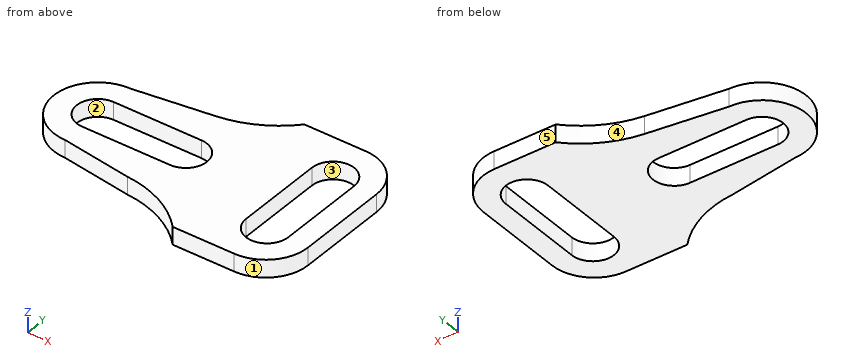
from build123d import *

# Parameters (mm, degrees)
BOSS_EXTRUDE1_DEPTH = 50


with BuildPart() as part:
    # Sketch1 → Boss-Extrude1 (new body)
    with BuildSketch(Plane.XY):
        with BuildLine():
            Line((-175, 353.543476539), (0, 353.543476539))
            ThreePointArc((0, 353.543476539), (84.852813742, 318.396290281), (120, 233.543476539))
            Line((120, 233.543476539), (120, -26.456523461))
            ThreePointArc((120, -26.456523461), (84.852813742, -111.309337204), (0, -146.456523461))
            Line((0, -146.456523461), (-175, -146.456523461))
            ThreePointArc((-175, -146.456523461), (-265.915006149, -79.830220617), (-375, -51.456523461))
            Line((-375, -51.456523461), (-575, -21.456523461))
            ThreePointArc((-575, -21.456523461), (-700, 103.543476539), (-575, 228.543476539))
            Line((-575, 228.543476539), (-355.89794699, 258.543476539))
            ThreePointArc((-355.89794699, 258.543476539), (-257.111916312, 290.168144661), (-175, 353.543476539))
        make_face()
        with BuildLine():
            Line((60, 228.543476539), (60, -21.456523461))
            ThreePointArc((60, -21.456523461), (0, -81.456523461), (-60, -21.456523461))
            Line((-60, -21.456523461), (-60, 228.543476539))
            ThreePointArc((-60, 228.543476539), (0, 288.543476539), (60, 228.543476539))
        make_face(mode=Mode.SUBTRACT)
        with BuildLine():
            Line((-325, 43.543476539), (-575, 43.543476539))
            ThreePointArc((-575, 43.543476539), (-635, 103.543476539), (-575, 163.543476539))
            Line((-575, 163.543476539), (-325, 163.543476539))
            ThreePointArc((-325, 163.543476539), (-265, 103.543476539), (-325, 43.543476539))
        make_face(mode=Mode.SUBTRACT)
    extrude(amount=BOSS_EXTRUDE1_DEPTH)


solid = part.part
Input: part model. Units: mm. Frame: model coordinates. Face numbers are marked on the shaded views. A direction names the side the tool comes from. Round coordinates to 2 decimals unless told otherwise and drop trailing zeros. Order: outer loops, then holes, each group sorted by start corner. A loop starts at its lowest first (then second) coordinate and runs counter-clockwise, first axis right, second up. Notation, with made-up numbers: (16.25, -34.5) - (45.25, -34.5) arc R28 cw to (45.25, -6.5) - close; hole circle Ø6 at (46.5, -35.5). An arc over 180 degrees is marked (long way). Answer as a JSON object with one key per item and string values. Group by question number.
(1) Reachability of the marked faces 1 and 2 from +Z, -Z, +X, -X, +Y, -Y: full face, straight path, thin tool, end or side. Return the list, or none.
(2) Pin query (flat end, axial travel): P1, Ø1, axis at x = -600, z = 18.5, coming from the +Y side; P2, Ø25, axis at y = 166, z = 14.5, coming from the -X side; P3, Ø4, axis at x = -506, z = 26, coming from the +Y side (3 decimals); P4, Ø2, axis at x = -173.5, y = -54.5, coming from the -Z side. Return the tip coordinate at first contact, or that it passes through.
(3) Cut plane B-B (y = 218). Return loops of the section in (x, z).
(4) Draft query along X for the marked faces 3, 4 and 5. Return one class per face: released by +X, released by -X, zero draft, split by the parting line, or undercut.
(5) Material intervals for probe 1 along X at (y, z) = (127, 16.5); probe 2 along X at (y, z) = (187, 30.5); probe 3 along X at (y, z) = (-6.5, 25.5), sorted ascending. Write a range as from..to.
(6) Cut plane A-A (x = -478). Return loops of the section in (y, z), then the cut area to 3 significant figures.
(7) Cut plane C-C (z = 10). Return loops of the section in (x, y), then the cut area to 3 significant figures.
(8) Cut plane D-D (y = 108). Return loops of the section in (x, z).
Here are the results:
{
 "1": {"face 1": "+Z, -Z, +X, -Y", "face 2": "+Z, -Z"},
 "2": {"P1": "stops at y = 226.12", "P2": "stops at x = -689.58", "P3": "stops at y = 238.265", "P4": "stops at z = 0"},
 "3": {"outline": "(-625.25, 0) - (-60, 0) - (-60, 50) - (-625.25, 50) - close; (60, 0) - (120, 0) - (120, 50) - (60, 50) - close"},
 "4": {"face 3": "undercut", "face 4": "released by -X", "face 5": "zero draft"},
 "5": {"probe 1": "x = -697.78..-630.22, -269.78..-60, 60..120", "probe 2": "x = -668.06..-60, 60..120", "probe 3": "x = -634.29..-60, 60..120"},
 "6": {"outline": "(-36.01, 0) - (43.54, 0) - (43.54, 50) - (-36.01, 50) - close; (163.54, 0) - (241.82, 0) - (241.82, 50) - (163.54, 50) - close", "area": "7,890 mm^2"},
 "7": {"outline": "(-575, -21.46) - (-375, -51.46) arc R300 cw to (-175, -146.46) - (0, -146.46) arc R120 ccw to (120, -26.46) - (120, 233.54) arc R120 ccw to (0, 353.54) - (-175, 353.54) arc R300 cw to (-355.9, 258.54) - (-575, 228.54) arc R125 ccw to start; hole (-575, 43.54) - (-325, 43.54) arc R60 ccw to (-325, 163.54) - (-575, 163.54) arc R60 ccw to start; hole (-60, -21.46) arc R60 ccw to (60, -21.46) - (60, 228.54) arc R60 ccw to (-60, 228.54) - close", "area": "213,000 mm^2"},
 "8": {"outline": "(-699.92, 0) - (-634.83, 0) - (-634.83, 50) - (-699.92, 50) - close; (-265.17, 0) - (-60, 0) - (-60, 50) - (-265.17, 50) - close; (60, 0) - (120, 0) - (120, 50) - (60, 50) - close"}
}
